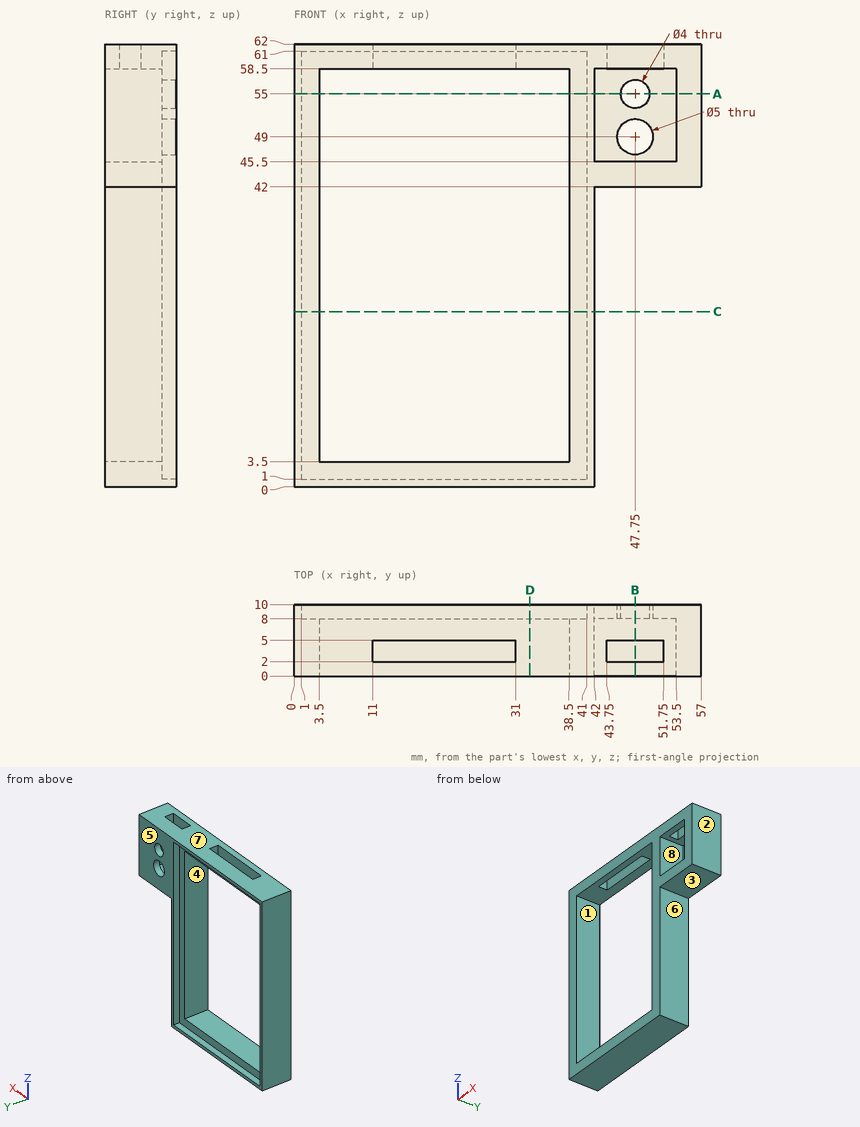
Study the drawing (mm; zero at the part's minimum x, y, z) and answer. A direction names the side the tool comes from. Round coordinates to 2 decimals unless told otherwise and drop trailing zeros. Loops run counter-clockwise (first coordinate to the right, second up) from the corner with the lowest first, then second, coordinate; pieces in that order, holes last. Notation, with made-up numbers: (23.5, -29) - (53.5, -29) arc R20 ccw to (53.5, -12) - close; hole circle Ø6 at (-26.75, -0.75). An arc over 180 degrees is marked (long way). Use one line per item in the form item = value. Start each with the question number.
1. The part is cut by section C-C on z = 24.5. Determine the outline of the cut face in (x, y), then the cut area to 3 significant figures.
2. Given pin 1 Ø1 at (x, z) = (17, 60) entering from +Y; pin 2 Ø3 at (x, y) = (50, 4) entering from -Z; pin 3 Ø6 at (x, z) = (49, 55) entering from -Y, each flat-ended and moving along its own axis, determine where each tip first touches the part or whether it passes through.
3. Consider line 1 (X direction, y = 3, z = 56); line 2 (X direction, y = 9.55, z = 49); line 3 (Z direction, x = 47.75, y = 9.1). Determine where each line is inside the solid, lowest interval first. Write a range as [from, to].
4. The part is cut by section D-D on x = 33. Determine the outline of the cut face in (y, z), then the cut area to 3 significant figures.
5. A tool of negligible diameter and unlimited length cuts with its end or side. For the marked faces 4, 5, 6, 7 and 8, from which of +Z, -Z, +X, -X, +Y, -Y can it reach the whole face along a straight path? Write none if from no direction.
6. The part is cut by section A-A on z = 55. Determine the outline of the cut face in (x, y), then the cut area to 3 significant figures.
7. For a pull along X with two mould halves and no side action, classify the marked faces 1, 2 and 3 as pulls with the +X half, pulls with the -X half, needs draft (parallel to the pull), parting line crosses it, or undercut.
8. The part is cut by section B-B on x = 47.75. Determine the outline of the cut face in (y, z), then the cut area to 3 significant figures.
Geometry check:
q1.outline = (0, 0) - (3.5, 0) - (3.5, 8) - (1, 8) - (1, 10) - (0, 10) - close; (38.5, 0) - (42, 0) - (42, 10) - (41, 10) - (41, 8) - (38.5, 8) - close
q1.area = 60.0 mm^2
q2.pin_1 = 8
q2.pin_2 = 42
q2.pin_3 = 8
q3.line_1 = [0, 3.5], [38.5, 42], [53.5, 57]
q3.line_2 = [0, 1], [41, 45.25], [50.25, 57]
q3.line_3 = [42, 46.5], [51.5, 53], [57, 62]
q4.outline = (0, 0) - (10, 0) - (10, 1) - (8, 1) - (8, 3.5) - (0, 3.5) - close; (0, 58.5) - (8, 58.5) - (8, 61) - (10, 61) - (10, 62) - (0, 62) - close
q4.area = 60.0 mm^2
q5.face_4 = +Y, -Y
q5.face_5 = +Z, -Z, +X, -X, +Y
q5.face_6 = -Z, +X, +Y, -Y
q5.face_7 = +Z, +X, -X, +Y, -Y
q5.face_8 = -Y
q6.outline = (0, 0) - (3.5, 0) - (3.5, 8) - (1, 8) - (1, 10) - (0, 10) - close; (38.5, 0) - (42, 0) - (42, 8) - (45.75, 8) - (45.75, 10) - (41, 10) - (41, 8) - (38.5, 8) - close; (49.75, 8) - (53.5, 8) - (53.5, 0) - (57, 0) - (57, 10) - (49.75, 10) - close
q6.area = 110 mm^2
q7.face_1 = undercut
q7.face_2 = pulls with the +X half
q7.face_3 = needs draft
q8.outline = (0, 42) - (10, 42) - (10, 46.5) - (8, 46.5) - (8, 45.5) - (0, 45.5) - close; (0, 58.5) - (2, 58.5) - (2, 62) - (0, 62) - close; (5, 58.5) - (8, 58.5) - (8, 57) - (10, 57) - (10, 62) - (5, 62) - close; (8, 51.5) - (10, 51.5) - (10, 53) - (8, 53) - close
q8.area = 67.5 mm^2
